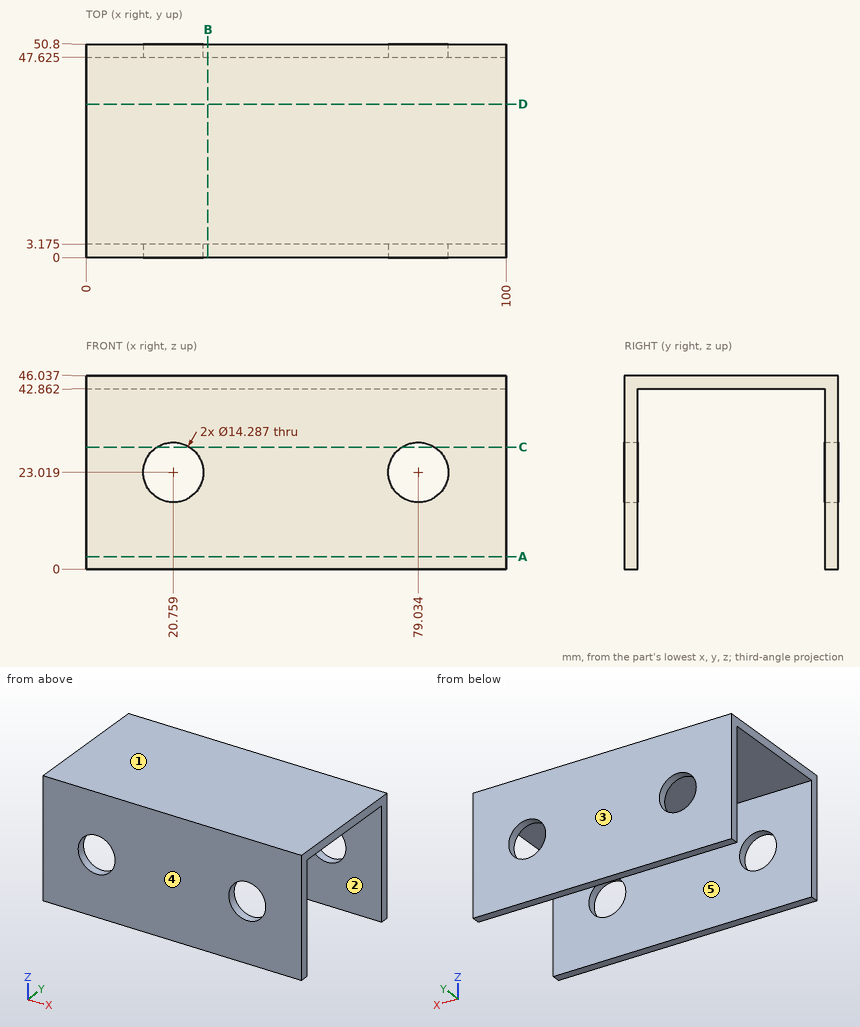
Drawing for the job (mm, zero at the part's lowest x, y, z). A direction names the side the tool comes from. Coordinates: 2 decimals unless noted, no trailing zeros. Loops run counter-clockwise (first coordinate to the right, second up) from the corner with the lowest first, then second, coordinate; pieces in that order, holes last. Notation, with made-up numbers: (-6.75, 4.5) - (37.25, 4.5) arc R17 cw to (37.25, 35.5) - close; hole circle Ø6 at (-35, -26.5). An arc over 180 degrees is marked (long way). Return JSON: item names as keys, results as strings.
1. Band-saw the part on B-B (x = 29). Give the cut face in (y, z) (1 decimal).
Result:
{"outline": "(0, 0) - (3.2, 0) - (3.2, 42.9) - (47.6, 42.9) - (47.6, 0) - (50.8, 0) - (50.8, 46) - (0, 46) - close"}
2. 3-axis set-ups, long thin cutter, end or side, ignore diameter. For the marked faces 1 and 2: which of +Z, -Z, +X, -X, +Y, -Y reach the whole face in a straight line?
Result:
{"face 1": "+Z, +X, -X, +Y, -Y", "face 2": "-Z, +X, -X"}
3. Band-saw the part on C-C (z = 29). Give the cut face in (x, y) (1 decimal).
Result:
{"outline": "(0, 0) - (16.9, 0) - (16.9, 3.2) - (0, 3.2) - close; (0, 47.6) - (16.9, 47.6) - (16.9, 50.8) - (0, 50.8) - close; (24.7, 0) - (75.1, 0) - (75.1, 3.2) - (24.7, 3.2) - close; (24.7, 47.6) - (75.1, 47.6) - (75.1, 50.8) - (24.7, 50.8) - close; (82.9, 0) - (100, 0) - (100, 3.2) - (82.9, 3.2) - close; (82.9, 47.6) - (100, 47.6) - (100, 50.8) - (82.9, 50.8) - close"}
4. Mould opens along Y. For the marked faces 3, 4 and 5 say: released by +Y, released by -Y, zero draft, split by the parting line, or undercut.
Result:
{"face 3": "released by +Y", "face 4": "released by -Y", "face 5": "undercut"}
5. Band-saw the part on A-A (z = 3). Give the cut face in (x, y) (1 decimal), and give its area (3 significant figures).
Result:
{"outline": "(0, 0) - (100, 0) - (100, 3.2) - (0, 3.2) - close; (0, 47.6) - (100, 47.6) - (100, 50.8) - (0, 50.8) - close", "area": "635 mm2"}
6. Band-saw the part on D-D (y = 36.5). Give the cut face in (x, z).
Result:
{"outline": "(0, 42.86) - (100, 42.86) - (100, 46.04) - (0, 46.04) - close"}
7. Probe L1, parallel to Y at x = 19, z = 42 (1 decimal); L2, parallel to Z at x = 9, y = 36. List the from-to ranges inside material, lowest first. Write a range as from..to.
Result:
{"L1": "y = 0..3.2, 47.6..50.8", "L2": "z = 42.86..46.04"}
8. Drop flat-ended pins along their axis: pin 1 (23 mm diameter, centred on x = 20.76, z = 23.02, fed in from -Y); pin 2 (4 mm diameter, centred on x = 55, y = 17.5, fed in from -Z). Give the stop position or say it passes through.
Result:
{"pin 1": "stops at y = 0", "pin 2": "stops at z = 42.86"}
